```python
from build123d import *

# Parameters (mm, degrees)
ESQUISSE1_R             = 50
BOSS_EXTRU_3_DEPTH      = 20
ESQUISSE2_R             = 68.25
ENL_V_MAT_EXTRU_9_DEPTH = 10


with BuildPart() as part:
    # Esquisse1 → Boss.-Extru.3 (new body)
    with BuildSketch(Plane.XY):
        with BuildLine():
            ThreePointArc((52.958333333, 53.107578843), (28.652500648, 69.311140566), (0, 75))
            ThreePointArc((0, 75), (-28.652500648, 69.311140566), (-52.958333333, 53.107578843))
            ThreePointArc((-52.958333333, 53.107578843), (-91.362529225, 32.640861336), (-134.666666667, 36.944402673))
            ThreePointArc((-134.666666667, 36.944402673), (-167.842344673, 35.800149952), (-188.729833462, 10))
            Line((-188.729833462, 10), (-172.912878475, 10))
            ThreePointArc((-172.912878475, 10), (-125, 0), (-172.912878475, -10))
            Line((-172.912878475, -10), (-188.729833462, -10))
            ThreePointArc((-188.729833462, -10), (-167.842344673, -35.800149952), (-134.666666667, -36.944402673))
            ThreePointArc((-134.666666667, -36.944402673), (-91.362529225, -32.640861336), (-52.958333333, -53.107578843))
            ThreePointArc((-52.958333333, -53.107578843), (0, -75), (52.958333333, -53.107578843))
            ThreePointArc((52.958333333, -53.107578843), (91.362529225, -32.640861336), (134.666666667, -36.944402673))
            ThreePointArc((134.666666667, -36.944402673), (167.842344673, -35.800149952), (188.729833462, -10))
            Line((188.729833462, -10), (172.912878475, -10))
            ThreePointArc((172.912878475, -10), (125, 0), (172.912878475, 10))
            Line((172.912878475, 10), (188.729833462, 10))
            ThreePointArc((188.729833462, 10), (167.842344673, 35.800149952), (134.666666667, 36.944402673))
            ThreePointArc((134.666666667, 36.944402673), (91.362529225, 32.640861336), (52.958333333, 53.107578843))
        make_face()
        Circle(ESQUISSE1_R, mode=Mode.SUBTRACT)
    extrude(amount=BOSS_EXTRU_3_DEPTH)

    # Esquisse2 → Enlèv. mat.-Extru.9 (cut)
    with BuildSketch(Plane.XY):
        Circle(ESQUISSE2_R)
    extrude(amount=ENL_V_MAT_EXTRU_9_DEPTH, mode=Mode.SUBTRACT)


solid = part.part
```
The listing builds one solid part. Answer for the finished solid, in the listing's coordinates (mm). A direction names the side the tool comes from. Give positions to 0.01 mm unless a question says otherwise; leave off trailing zeros. Write each loop counter-clockwise with the first axis right and the second up, starting at its lowest first coordinate (ties: lowest second). Pieces come first, ordered by that corner, then holes. Notation, with made-up numbers: (77, 45.25) - (89, 45.25) arc R14 cw to (89, 63.25) - close; hole circle Ø3 at (27, 63.5). An arc over 180 degrees is marked (long way). Use one line per item in the form item = value. Start each with the question number.
1) A tool of negligible diameter and unlimited length cuts with its end or side. For faces 1 (the face through (181, -10, 10)), 2 (the face through (47.69, 15.02, 14.93)), 3 (the face through (36.69, 57.55, 4.93)), 4 (the face through (-181, -10, 10)), from which of +Z, -Z, +X, -X, +Y, -Y can it reach the whole face along a straight path? Write none if from no direction.
2) Consider line 1 along Y through (x, z) = (0, 12.5); line 2 along Y through (x, z) = (0, 6); line 3 along Z through (x, y) = (-46, 21.5). Determine where each line is inside the solid, lowest interval first. Write a range as from..to.
3) Flat-ended cylindrical pins translate along their axes: pin 1 Ø10 at (x, z) = (138.5, 5.5) entering from +Y; pin 2 Ø4 at (x, z) = (66, 13) entering from -Y; pin 3 Ø5 at (y, z) = (55, 4) entering from +X. Find the tip coordinate at first contact, or state that the pin passes through.
4) Find section C-C on z = 6. Determine the outline of the cut face in (x, y).
5) Find section B-B on x = -22. Determine the outline of the cut face in (y, z).
6) Find section A-A on y = 0. Determine the outline of the cut face in (x, z).
7) Find section D-D on x = -150. Determine the outline of the cut face in (y, z), plus the area to 3 significant figures.
Geometry results:
q1.face_1 = +Z, -Z, +X
q1.face_2 = +Z, -Z
q1.face_3 = -Z
q1.face_4 = +Z, -Z, -X
q2.line_1 = -75..-50, 50..75
q2.line_2 = -75..-68.25, 68.25..75
q2.line_3 = 10..20
q3.pin_1 = 39.47
q3.pin_2 = -44.02
q3.pin_3 = 53.57
q4.outline = (-188.73, -10) arc R40 ccw to (-134.67, -36.94) arc R75 cw to (-52.96, -53.11) arc R75 ccw to (52.96, -53.11) arc R75 cw to (134.67, -36.94) arc R40 ccw to (188.73, -10) - (172.91, -10) arc R25 cw (long way) to (172.91, 10) - (188.73, 10) arc R40 ccw to (134.67, 36.94) arc R75 cw to (52.96, 53.11) arc R75 ccw to (-52.96, 53.11) arc R75 cw to (-134.67, 36.94) arc R40 ccw to (-188.73, 10) - (-172.91, 10) arc R25 cw (long way) to (-172.91, -10) - close; hole circle Ø136.5 at (0, 0)
q5.outline = (-71.7, 0) - (-64.61, 0) - (-64.61, 10) - (-44.9, 10) - (-44.9, 20) - (-71.7, 20) - close; (44.9, 10) - (64.61, 10) - (64.61, 0) - (71.7, 0) - (71.7, 20) - (44.9, 20) - close
q6.outline = (-125, 0) - (-68.25, 0) - (-68.25, 10) - (-50, 10) - (-50, 20) - (-125, 20) - close; (50, 10) - (68.25, 10) - (68.25, 0) - (125, 0) - (125, 20) - (50, 20) - close
q7.outline = (-40, 0) - (-25, 0) - (-25, 20) - (-40, 20) - close; (25, 0) - (40, 0) - (40, 20) - (25, 20) - close
q7.area = 600 mm2
